Read the model definition and answer for the solid it produces. Units are mm, in the model's axes. A direction names the side the tool comes from. Give positions to 0.01 mm unless a question says otherwise; leave off trailing zeros. Write each question's results on one line, items separated by ' | '.
from build123d import *

# Parameters (mm, degrees)
CYLINDER005_R            = 11.3
CYLINDER005_DEPTH        = 14.5
CYLINDER004_R            = 2.3
CYLINDER004_DEPTH        = 14.5
ARRAY_COUNT              = 4
CYLINDER003_R            = 8.3
CYLINDER003_DEPTH        = 14.5
CYLINDER002_R            = 12.3
CYLINDER002_DEPTH        = 14.5
CHAMFER_SIZE             = 0.5
CLONE001_PLACEMENT_ANGLE = 76


with BuildPart() as cylinder005:
    # Cylinder005 → Cylinder005 (new body)
    with BuildSketch(Plane.XY.offset(-1)):
        Circle(CYLINDER005_R)
    extrude(amount=CYLINDER005_DEPTH)


with BuildPart() as array:
    # Cylinder004 → Cylinder004 (new body)
    with BuildSketch(Plane(origin=(0, -5, 14), x_dir=(1, 0, 0), z_dir=(0, 0, 1))):
        Circle(CYLINDER004_R)
    extrude(amount=CYLINDER004_DEPTH)

    # Array: Array ×4 about axis
    array_axis = Axis((0, 0, 0), (0, 0, 1))


with BuildPart() as array_1:
    add(array.part)
    for i in range(1, ARRAY_COUNT):
        add(array.part.rotate(array_axis, i * 360 / ARRAY_COUNT))


with BuildPart() as cylinder003:
    # Cylinder003 → Cylinder003 (new body)
    with BuildSketch(Plane.XY.offset(14.5)):
        Circle(CYLINDER003_R)
    extrude(amount=CYLINDER003_DEPTH)


with BuildPart() as cup_compound_clone:
    # Cylinder002 → Cylinder002 (new body)
    with BuildSketch(Plane.XY):
        Circle(CYLINDER002_R)
    extrude(amount=CYLINDER002_DEPTH)

    # Cut002: cut Cylinder003
    add(cylinder003.part, mode=Mode.SUBTRACT)

    # Cut003: cut Array
    add(array_1.part, mode=Mode.SUBTRACT)

    # Cut004: cut Cylinder005
    add(cylinder005.part, mode=Mode.SUBTRACT)

    # Chamfer
    chamfer_edges = [cup_compound_clone.edges().sort_by_distance(p)[0] for p in [
        (-12.3, 0, 14.5),
    ]]
    chamfer(chamfer_edges, length=CHAMFER_SIZE)


with BuildPart() as cup_compound_clone_1:
    # Clone001 placement: moved
    add(cup_compound_clone.part.moved(Location((76, 24, 18))).rotate(Axis((76, 24, 18), (0, 1, 0)), CLONE001_PLACEMENT_ANGLE))


solid = cup_compound_clone_1.part
(1) The mould has two halves that part along X. Classify faces 1 (the face through (89.382, 17.6, 23.218)), 2 (the face through (76.868, 13.124, 14.52)), 3 (the face through (85.535, 27.695, 8.286)): pulls with the +X half, pulls with the -X half, needs draft (parallel to the pull), parting line crosses it, or undercut.
Conclusion:
face 1: undercut | face 2: pulls with the -X half | face 3: parting line crosses it
(2) Consider probe 1 along Y at (x, z) = (90, 21.5); probe 2 along Y at (x, z) = (76.75, 22); probe 3 along Y at (x, z) = (87.75, 20.5). Determine where each line is inside the solid, lowest interval first. Write a range as [from, to].
Conclusion:
probe 1: [12.13, 16.7], [21.3, 26.7], [31.3, 35.87] | probe 2: [12.27, 13.32], [34.68, 35.73] | probe 3: [11.71, 12.71], [35.29, 36.29]
(3) Each of these flat-tipped pins is pushed along its axis until it touches: pin 1 (6 mm diameter, centred on y = 24.5, z = 9, fed in from -X); pin 2 (10 mm diameter, centred on y = 14.5, z = 13.5, fed in from +X); pin 3 (5 mm diameter, centred on y = 29, z = 22, fed in from +X). Where does it stop, or does it pass through?
Conclusion:
pin 1: x = 78.63 | pin 2: x = 92.65 | pin 3: x = 90.26
(4) For faces 4 (the face through (89.06, 24.16, 21.42)), 5 (the face through (90.03, 24.17, 21.67)), determine the directions among +Z, -Z, +X, -X, +Y, -Y from which every point of the face is accessible in a straight line to the end or side of a thin tool.
Conclusion:
face 4: none | face 5: +Z, +X, +Y, -Y
